Here's how the part is built. I have some questions about the finished solid (model axes, mm). A direction names the side the tool comes from. Round coordinates to 2 decimals unless told otherwise and drop trailing zeros. Write each loop counter-clockwise with the first axis right and the second up, starting at its lowest first coordinate (ties: lowest second). Pieces come first, ordered by that corner, then holes. Notation, with made-up numbers: M -2.75,10 L 5.25,10 A13 cw 5.25,19 Z; hole C 75.25,79.5 d2. An arc over 180 degrees is marked long. Write item = value, one per line. Start each with the question number.
(1) On a 3-axis mill with a long thin cutter (end or side, diameter ignored), from which of +Z, -Z, +X, -X, +Y, -Y can I reach the whole of each face in a straight line? I mean faces 4 (the flat face through (-52.48, -14.06, 1.97)), 5 (the flat face through (-14.636, 23.327, 1.972)), 6 (the cylindrical face through (-49.65, -5.9, 1.97)), 7 (the flat face through (-24, 14, 4)), 8 (the flat face through (-68.55, -1.045, 1.972)). Say none if no direction works.
(2) I want a section at B-B (y = -5). List the corners of the cut face in (x, z) for me, and give its area (3 significant figures).
(3) Will this pin go through, and if not, where does the flat tip stop? pin 1 Ø1 at (x, z) = (-32.5, 0.5) entering from +Y.
(4) I want a section at C-C (x = -35.5). List the corners of the cut face in (y, z) for me, and give its area (3 significant figures).
(5) I want a section at D-D (x = 0). List the corners of the cut face in (y, z) for me.
(6) I need wall thicknesses on line 1 along X through (y, z) = (-3, 3.35); line 2 along X through (y, z) = (-3.5, 2.6); line 3 along Y through (x, z) = (0, 1.05). Which ranges of each line are inside material? Lowest first, please.
(7) If we mould it in two halves opening along Y, with no side actions, what happens to faces 1 (the cylindrical face through (31.802, 22.202, 1.972)), 2 (the cylindrical face through (-5.158, -3.955, 1.972)), 3 (the flat face through (-24, 14, 0))? For each: released by +Y, released by -Y, zero draft, split by the parting line, or undercut.
(8) I want a section at A-A (x = 25.5). List the corners of the cut face in (y, z) for me.
```python
from build123d import *

# Parameters (mm, degrees)
SKETCH_1_R             = 3
SKETCH_1_R_2           = 6.5
SM_BASE_FLANGE_1_DEPTH = 4
CHAMFER_2_SIZE         = 1.5


# Sheet-metal steps are written as plain solids
with BuildPart() as part:
    # Sketch 1 → Базовая кромка1 (new body)
    with BuildSketch(Plane.XY):
        with BuildLine():
            Line((-31.781350826, 25.798136577), (2.996060756, 20.785177891))
            ThreePointArc((2.996060756, 20.785177891), (4.303188162, 20.554380838), (5.593123802, 20.241466502))
            ThreePointArc((5.593123802, 20.241466502), (14.252686638, 20.246803625), (21.67545772, 24.706683273))
            ThreePointArc((21.67545772, 24.706683273), (31.84775804, 22.028007779), (24.127078994, 14.883631579))
            ThreePointArc((24.127078994, 14.883631579), (19.607693171, 13.67003856), (18.956512096, 9.036074875))
            ThreePointArc((18.956512096, 9.036074875), (4.632129423, -20.482758042), (-21, 0))
            ThreePointArc((-21, 0), (-35.5, 14.5), (-50, 0))
            ThreePointArc((-50, 0), (-49.640340933, -5.986363846), (-48.566537916, -11.88660569))
            ThreePointArc((-48.566537916, -11.88660569), (-48.457937157, -12.423224233), (-48.39294532, -12.966850618))
            Line((-48.39294532, -12.966850618), (-56.68245323, -15.188017568))
            Line((-56.68245323, -15.188017568), (-80.754558191, 13.5))
            Line((-80.754558191, 13.5), (-43.07213712, 24.940628339))
            ThreePointArc((-43.07213712, 24.940628339), (-37.473872446, 25.989921702), (-31.781350826, 25.798136577))
        make_face()
        with Locations((11.189842551, 14.585216118)):
            Circle(SKETCH_1_R, mode=Mode.SUBTRACT)
        Circle(SKETCH_1_R_2, mode=Mode.SUBTRACT)
        with Locations((26.026325977, 20.575104227)):
            Circle(SKETCH_1_R, mode=Mode.SUBTRACT)
    extrude(amount=SM_BASE_FLANGE_1_DEPTH)

    # Фаска2
    chamfer_2_edges = [part.edges().sort_by_distance(p)[0] for p in [
        (8.189842551, 14.585216118, 0),
    ]]
    chamfer(chamfer_2_edges, length=CHAMFER_2_SIZE)


solid = part.part
```
Returned:
q1.face_4 = +Z, -Z, -Y
q1.face_5 = +Z, -Z, +Y
q1.face_6 = +Z, -Z
q1.face_7 = +Z, +X, -X, +Y, -Y
q1.face_8 = +Z, -Z, -X, -Y
q2.outline = M -65.23,0 L -49.75,0 L -49.75,4 L -65.23,4 Z; M -20.4,0 L -4.15,0 L -4.15,4 L -20.4,4 Z; M 4.15,0 L 20.4,0 L 20.4,4 L 4.15,4 Z
q2.area = 192 mm²
q3.pin_1 = 25.94
q4.outline = M 14.5,0 L 26.06,0 L 26.06,4 L 14.5,4 Z
q4.area = 46.3 mm²
q5.outline = M -21,0 L -6.5,0 L -6.5,4 L -21,4 Z; M 6.5,0 L 21.22,0 L 21.22,4 L 6.5,4 Z
q6.line_1 = -66.91 to -49.91, -20.78 to -5.77, 5.77 to 20.78
q6.line_2 = -66.49 to -49.88, -20.71 to -5.48, 5.48 to 20.71
q6.line_3 = -21 to -6.5, 6.5 to 21.22
q7.face_1 = split by the parting line
q7.face_2 = undercut
q7.face_3 = zero draft
q8.outline = M 14.6,0 L 17.62,0 L 17.62,4 L 14.6,4 Z; M 23.53,0 L 26.55,0 L 26.55,4 L 23.53,4 Z
